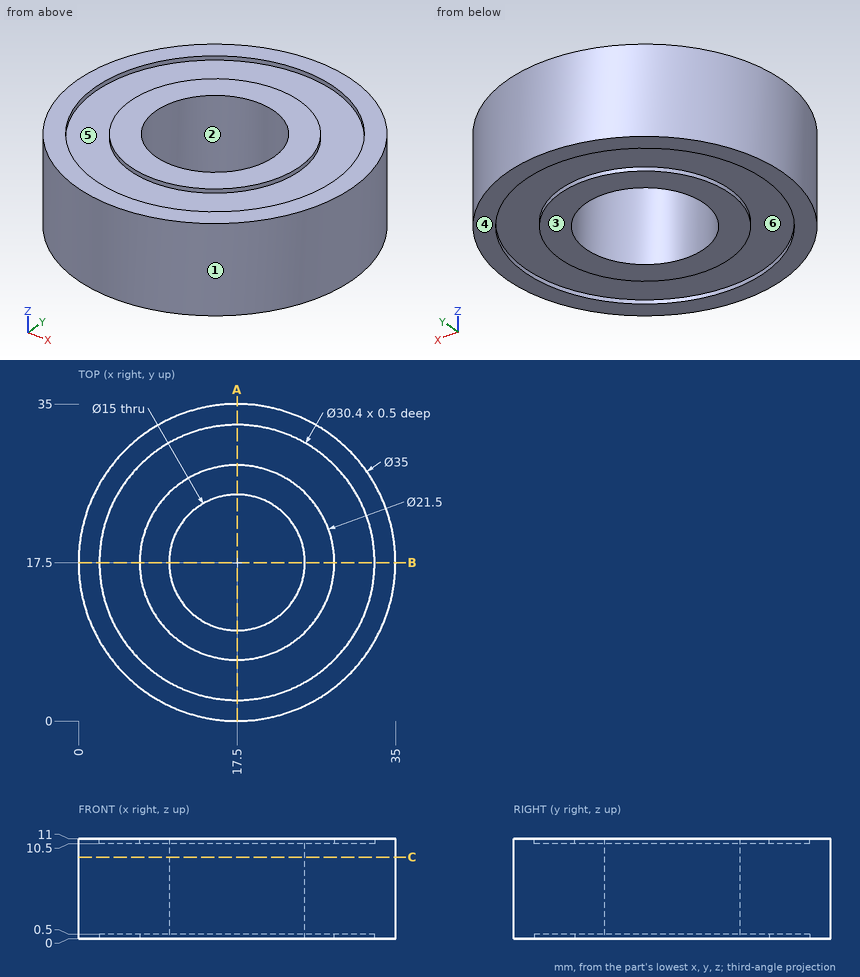
Source: three-view drawing plus pictorial views. Frame: mm from the lowest corner of the part. A direction names the side the tool comes from. Round coordinates to 2 decimals unless told otherwise and drop trailing zeros. Write each loop counter-clockwise with the first axis right and the second up, starting at its lowest first coordinate (ties: lowest second). Pieces come first, ordered by that corner, then holes. Notation, with made-up numbers: M 47,76.25 L 54,76.25 A28 ccw 54,99.25 Z; hole C 71.5,-0.5 d8. An arc over 180 degrees is marked long. Use CSV: the item, a comma, the result in double quotes. Start each with the question number.
Q1. First-contact query: P1, Ø6, axis at y = 28.5, z = 9.5, coming from the +X side; P2, Ø5, axis at x = 14, z = 8.5, coming from the +Y side; P3, Ø1, axis at y = 19, z = 9.5, coming from the -X side. Flat tips, straight axial feed; report the tip coordinate or a pass-through.
Q2. Pull-direction query (Y, two-part tool) for the marked faces 1, 2 and 3; classes: +Y half, -Y half, draft (parallel to the pull), parting line (faces both ways), or undercut.
Q3. Cut plane A-A on x = 17.5. Output: boundary loops of the cut face in (y, z).
Q4. Access query for the marked faces 4, 5 and 6. Directions: +Z, -Z, +X, -X, +Y, -Y. A direction counts if a zero-diameter tool reaches every point of the face in a straight line with its end or side. Return the directions, or none.
Q5. Cut plane C-C on z = 9. Output: boundary loops of the cut face in (x, y).
Q6. Line query: line 1 (Y direction, x = 17.5, z = 0.1); line 2 (Y direction, x = 17.5, z = 5); line 3 (X direction, y = 16.5, z = 6). Output: solid intervals per line, ascending. Write a range as from..to.
Results found:
1,P1,"x = 33.06"
1,P2,"y = 34.97"
1,P3,"x = 0.03"
2,face 1,"parting line"
2,face 2,"undercut"
2,face 3,"draft"
3,outline,"M 0,0 L 2.3,0 L 2.3,0.5 L 6.75,0.5 L 6.75,0 L 10,0 L 10,11 L 6.75,11 L 6.75,10.5 L 2.3,10.5 L 2.3,11 L 0,11 Z; M 25,0 L 28.25,0 L 28.25,0.5 L 32.7,0.5 L 32.7,0 L 35,0 L 35,11 L 32.7,11 L 32.7,10.5 L 28.25,10.5 L 28.25,11 L 25,11 Z"
4,face 4,"-Z, +X, -X, +Y, -Y"
4,face 5,"+Z"
4,face 6,"-Z"
5,outline,"C 17.5,17.5 d35; hole C 17.5,17.5 d15"
6,line 1,"0..2.3, 6.75..10, 25..28.25, 32.7..35"
6,line 2,"0..10, 25..35"
6,line 3,"0.03..10.07, 24.93..34.97"
